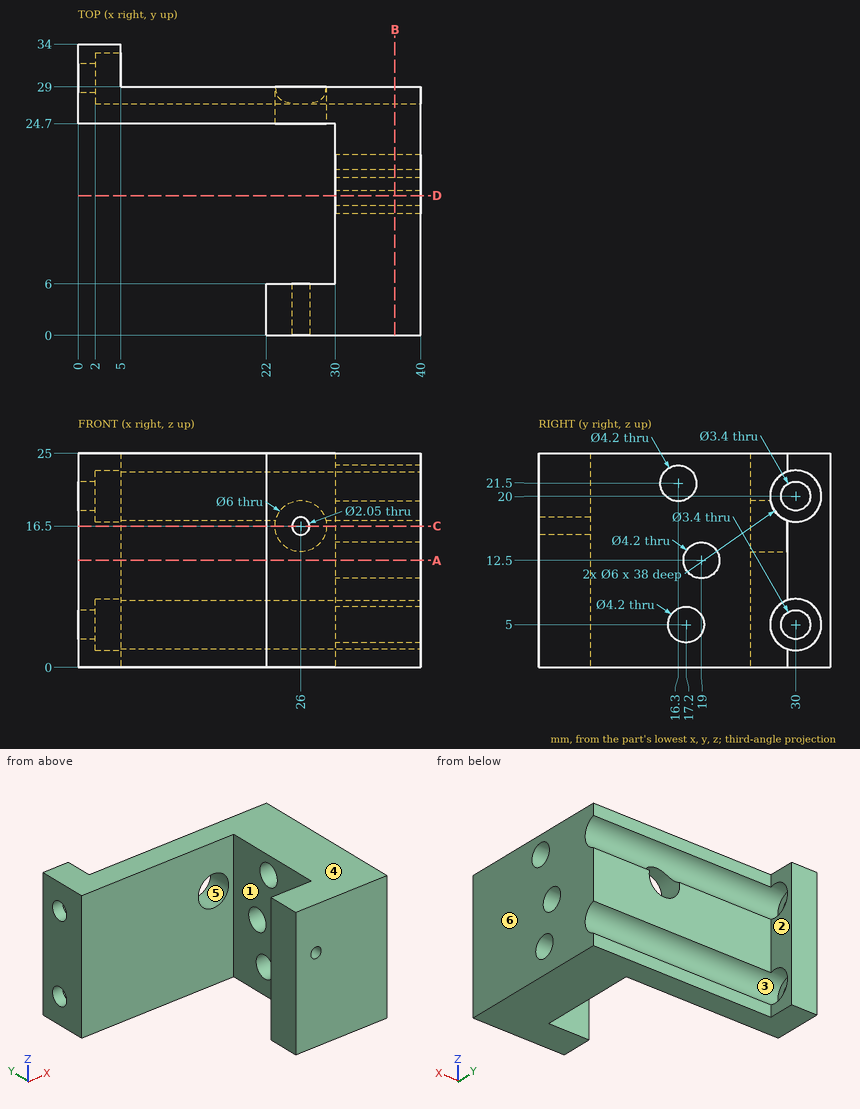
Source: three-view drawing plus pictorial views. Frame: mm from the lowest corner of the part. A direction names the side the tool comes from. Coordinates: 2 decimals unless noted, no trailing zeros. Order: outer loops, then holes, each group sorted by start corner. A loop starts at its lowest first (then second) coordinate and runs counter-clockwise, first axis right, second up. Notation, with made-up numbers: M 83,-12.5 L 122,-12.5 A25 ccw 122,20.5 Z; hole C -19,57.5 d2. An arc over 180 degrees is marked long. One line per question, with ' | ' between items. Start each with the question number.
Item 1: Cut plane D-D, the plane y = 16.3. Return the cut outline in (x, z).
Item 2: Set-up query: the marked faces 1, 2 and 3. Return all of +Z, -Z, +X, -X, +Y, -Y with unobstructed straight access to the full face (end or side cutting, diameter ignored); none if empty.
Item 3: Cut plane B-B, the plane x = 37. Return the cut outline in (y, z).
Item 4: Cut plane A-A, the plane z = 12.5. Return the cut outline in (x, y), then the cut area to 3 significant figures.
Item 5: Draft query along X for the marked faces 4, 5 and 6. Return one class per face: released by +X, released by -X, zero draft, split by the parting line, or undercut.
Item 6: Pin query (flat end, axial travel): pin 1 Ø2.5 at (y, z) = (30, 20) entering from +X; pin 2 Ø3 at (x, z) = (19.5, 10.5) entering from +Y; pin 3 Ø5 at (y, z) = (17.5, 16.5) entering from -X; pin 4 Ø5 at (x, z) = (26, 16.5) entering from +Y. Return the tip coordinate at first contact, or that it passes through.
Item 7: Ray query, probe 1 along Y at (x, z) = (1, 20); probe 2 along Y at (x, z) = (23.5, 20.25); probe 3 along X at (y, z) = (14.5, 4.5). Return the intervals inside material, ascending. Write a range as [from, to].
Item 8: Cut plane C-C, the plane z = 16.5. Return the cut outline in (x, y) (3 decimals).
A:
1) outline: M 30,0 L 40,0 L 40,3.1 L 30,3.1 Z; M 30,6.9 L 40,6.9 L 40,19.4 L 30,19.4 Z; M 30,23.6 L 40,23.6 L 40,25 L 30,25 Z
2) face 1: +Z, -Z, -X | face 2: +Z, -Z, +X, +Y | face 3: +X
3) outline: M 0,0 L 29,0 L 29,2.17 A3 cw 29,7.83 L 29,17.17 A3 cw 29,22.83 L 29,25 L 0,25 Z; hole C 16.3,21.5 d4.2; hole C 17.2,5 d4.2; hole C 19,12.5 d4.2
4) outline: M 0,24.7 L 30,24.7 L 30,21.1 L 40,21.1 L 40,29 L 5,29 L 5,34 L 0,34 Z; M 22,0 L 40,0 L 40,16.9 L 30,16.9 L 30,6 L 22,6 Z | area: 450 mm2
5) face 4: zero draft | face 5: undercut | face 6: released by +X
6) pin 1: passes through | pin 2: stops at y = 29 | pin 3: stops at x = 30 | pin 4: stops at y = 6
7) probe 1: y = [24.7, 28.3], [31.7, 34] | probe 2: y = [0, 6], [24.7, 27.01] | probe 3: x = [30, 40]
8) outline: M 0,24.7 L 23,24.7 L 23,29 L 5,29 L 5,34 L 0,34 Z; M 22,0 L 24.975,0 L 24.975,6 L 22,6 Z; M 27.025,0 L 40,0 L 40,29 L 29,29 L 29,24.7 L 30,24.7 L 30,6 L 27.025,6 Z
